```python
from build123d import *

# Parameters (mm, degrees)
F0_R      = 9.525
F1_DEPTH  = 25.4
F3_DEPTH  = 50
F5_DEPTH  = 25.401
F6_DEPTH  = 9.398
F7_DEPTH  = 12.7
F8_DEPTH  = 11.0998
F10_DEPTH = 9.525
F11_R     = 0.508


# Not quite as in the source:
# - an extrude ends at something that could not be found from the text; its depth is read off the source's solid


with BuildPart() as f1:
    # F0 (on Front) → F1 (new body)
    with BuildSketch(Plane.XZ):
        Circle(F0_R)
    extrude(amount=F1_DEPTH)

    # F2 (on Front) → F3 (cut, through all)
    with BuildSketch(Plane.XZ):
        with BuildLine():
            ThreePointArc((4.7625, 0), (3.3675960454, 3.3675960454), (0, 4.7625))
            ThreePointArc((0, 4.7625), (-3.3675960454, 3.3675960454), (-4.7625, 0))
            ThreePointArc((-4.7625, 0), (-3.3675960454, -3.3675960454), (0, -4.7625))
            ThreePointArc((0, -4.7625), (3.3675960454, -3.3675960454), (4.7625, 0))
        make_face()
    extrude(amount=-F3_DEPTH, mode=Mode.SUBTRACT)

    # F4 (on face) → F5 (cut, through all)
    with BuildSketch(Plane(origin=(0, 0, 0), x_dir=(-1, 0, 0), z_dir=(0, 1, 0))):
        with BuildLine():
            ThreePointArc((-4.7625, 0), (-3.3675960454, -3.3675960454), (0, -4.7625))
            ThreePointArc((0, -4.7625), (3.3675960454, -3.3675960454), (4.7625, 0))
            ThreePointArc((4.7625, 0), (3.3675960454, 3.3675960454), (0, 4.7625))
            ThreePointArc((0, 4.7625), (-3.3675960454, 3.3675960454), (-4.7625, 0))
        make_face()
    extrude(amount=-F5_DEPTH, mode=Mode.SUBTRACT)

    # F2 (on Front) → F6 (cut)
    with BuildSketch(Plane.XZ):
        with BuildLine():
            Line((4.7625, 0), (4.7625, 4.7625))
            Line((4.7625, 4.7625), (0, 4.7625))
            ThreePointArc((0, 4.7625), (3.3675960454, 3.3675960454), (4.7625, 0))
        make_face()
        with BuildLine():
            ThreePointArc((-4.7625, 0), (-3.3675960454, 3.3675960454), (0, 4.7625))
            Line((0, 4.7625), (-4.7625, 4.7625))
            Line((-4.7625, 4.7625), (-4.7625, 0))
        make_face()
        with BuildLine():
            ThreePointArc((4.7625, 0), (3.3675960454, 3.3675960454), (0, 4.7625))
            ThreePointArc((0, 4.7625), (-3.3675960454, 3.3675960454), (-4.7625, 0))
            ThreePointArc((-4.7625, 0), (-3.3675960454, -3.3675960454), (0, -4.7625))
            ThreePointArc((0, -4.7625), (3.3675960454, -3.3675960454), (4.7625, 0))
        make_face()
        with BuildLine():
            Line((4.7625, -4.7625), (4.7625, 0))
            ThreePointArc((4.7625, 0), (3.3675960454, -3.3675960454), (0, -4.7625))
            Line((0, -4.7625), (4.7625, -4.7625))
        make_face()
        with BuildLine():
            ThreePointArc((0, -4.7625), (-3.3675960454, -3.3675960454), (-4.7625, 0))
            Line((-4.7625, 0), (-4.7625, -4.7625))
            Line((-4.7625, -4.7625), (0, -4.7625))
        make_face()
    extrude(amount=-F6_DEPTH, mode=Mode.SUBTRACT)

    # F2 (on Front) → F7 (cut)
    with BuildSketch(Plane.XZ):
        with BuildLine():
            Line((4.7625, 0), (4.7625, 4.7625))
            Line((4.7625, 4.7625), (0, 4.7625))
            ThreePointArc((0, 4.7625), (3.3675960454, 3.3675960454), (4.7625, 0))
        make_face()
        with BuildLine():
            ThreePointArc((-4.7625, 0), (-3.3675960454, 3.3675960454), (0, 4.7625))
            Line((0, 4.7625), (-4.7625, 4.7625))
            Line((-4.7625, 4.7625), (-4.7625, 0))
        make_face()
        with BuildLine():
            ThreePointArc((4.7625, 0), (3.3675960454, 3.3675960454), (0, 4.7625))
            ThreePointArc((0, 4.7625), (-3.3675960454, 3.3675960454), (-4.7625, 0))
            ThreePointArc((-4.7625, 0), (-3.3675960454, -3.3675960454), (0, -4.7625))
            ThreePointArc((0, -4.7625), (3.3675960454, -3.3675960454), (4.7625, 0))
        make_face()
        with BuildLine():
            Line((4.7625, -4.7625), (4.7625, 0))
            ThreePointArc((4.7625, 0), (3.3675960454, -3.3675960454), (0, -4.7625))
            Line((0, -4.7625), (4.7625, -4.7625))
        make_face()
        with BuildLine():
            ThreePointArc((0, -4.7625), (-3.3675960454, -3.3675960454), (-4.7625, 0))
            Line((-4.7625, 0), (-4.7625, -4.7625))
            Line((-4.7625, -4.7625), (0, -4.7625))
        make_face()
    extrude(amount=-F7_DEPTH, mode=Mode.SUBTRACT)

    # F2 (on Front) → F8 (cut)
    with BuildSketch(Plane.XZ):
        with BuildLine():
            Line((4.7625, 0), (4.7625, 4.7625))
            Line((4.7625, 4.7625), (0, 4.7625))
            ThreePointArc((0, 4.7625), (3.3675960454, 3.3675960454), (4.7625, 0))
        make_face()
        with BuildLine():
            ThreePointArc((-4.7625, 0), (-3.3675960454, 3.3675960454), (0, 4.7625))
            Line((0, 4.7625), (-4.7625, 4.7625))
            Line((-4.7625, 4.7625), (-4.7625, 0))
        make_face()
        with BuildLine():
            ThreePointArc((4.7625, 0), (3.3675960454, 3.3675960454), (0, 4.7625))
            ThreePointArc((0, 4.7625), (-3.3675960454, 3.3675960454), (-4.7625, 0))
            ThreePointArc((-4.7625, 0), (-3.3675960454, -3.3675960454), (0, -4.7625))
            ThreePointArc((0, -4.7625), (3.3675960454, -3.3675960454), (4.7625, 0))
        make_face()
        with BuildLine():
            Line((4.7625, -4.7625), (4.7625, 0))
            ThreePointArc((4.7625, 0), (3.3675960454, -3.3675960454), (0, -4.7625))
            Line((0, -4.7625), (4.7625, -4.7625))
        make_face()
        with BuildLine():
            ThreePointArc((0, -4.7625), (-3.3675960454, -3.3675960454), (-4.7625, 0))
            Line((-4.7625, 0), (-4.7625, -4.7625))
            Line((-4.7625, -4.7625), (0, -4.7625))
        make_face()
    extrude(amount=F8_DEPTH, mode=Mode.SUBTRACT)

    # F9 (on face) → F10 (cut)
    with BuildSketch(Plane.XZ.offset(25.4)):
        Polygon((3.65125, 6.3241505111), (-3.65125, 6.3241505111), (-7.3025, 0), (-3.65125, -6.3241505111), (3.65125, -6.3241505111), (7.3025, 0), align=None)
    extrude(amount=-F10_DEPTH, mode=Mode.SUBTRACT)

    # F11
    f11_edges = [f1.edges().sort_by_distance(p)[0] for p in [
        (-9.525, -25.4, 0),
        (-5.476875, -25.4, 3.162075),
        (0, -25.4, 6.324151),
        (5.476875, -25.4, 3.162075),
        (-5.476875, -25.4, -3.162075),
        (0, -25.4, -6.324151),
        (5.476875, -25.4, -3.162075),
    ]]
    fillet(f11_edges, radius=F11_R)


solid = f1.part
```
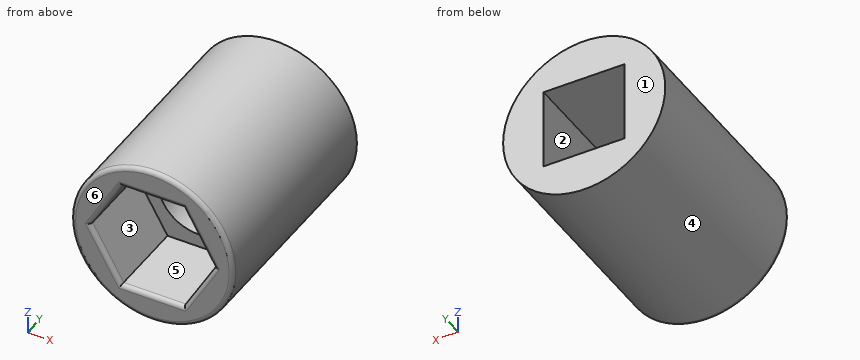
Work out the finished part from the listing and answer in its coordinate system (mm). Face numbers are marked on the shaded views. A direction names the side the tool comes from. Round coordinates to 2 decimals unless told otherwise and drop trailing zeros. Write each question's results on one line, items separated by ' | '.
1) Consider line 1 along Z through (x, y) = (4.5, -22.5); line 2 along Z through (x, y) = (-4.25, -10.5); line 3 along X through (y, z) = (-6, -2.5). Determine where each line is inside the solid, lowest interval first. Write a range as [from, to].
Findings:
line 1: z = [-8.39, -4.85], [4.85, 8.39] | line 2: z = [-8.52, -4.76], [4.76, 8.52] | line 3: x = [-9.19, -4.76], [4.76, 9.19]
2) Flat-ended cylindrical pins translate along their axes: pin 1 (5 mm diameter, centred on x = 2, z = -3.5, fed in from +Y); pin 2 (1.5 mm diameter, centred on x = -6, y = -16.5, fed in from +Z); pin 3 (1.4 mm diameter, centred on x = -2, z = 2.5, fed in from +Y); pin 4 (3 mm diameter, centred on x = 1.5, z = -4, fed in from -Y) (3 decimals). Find the tip coordinate at first contact, or state that the pin passes through.
Findings:
pin 1: stops at y = 0 | pin 2: stops at z = 7.95 | pin 3: passes through | pin 4: stops at y = -15.875
3) Which of the six approach directions +Z, -Z, +X, -X, +Y, -Y give full straight-line access (tool end or side, diameter ignored) to the marked faces 1, 2 and 3?
Findings:
face 1: +Z, -Z, +X, -X, +Y | face 2: +Y | face 3: -Y
4) For a pull along X with two mould halves and no side action, classify the marked faces 4, 5 and 6 as +X half, -X half, draft (parallel to the pull), parting line (faces both ways), or undercut.
Findings:
face 4: parting line | face 5: undercut | face 6: draft
